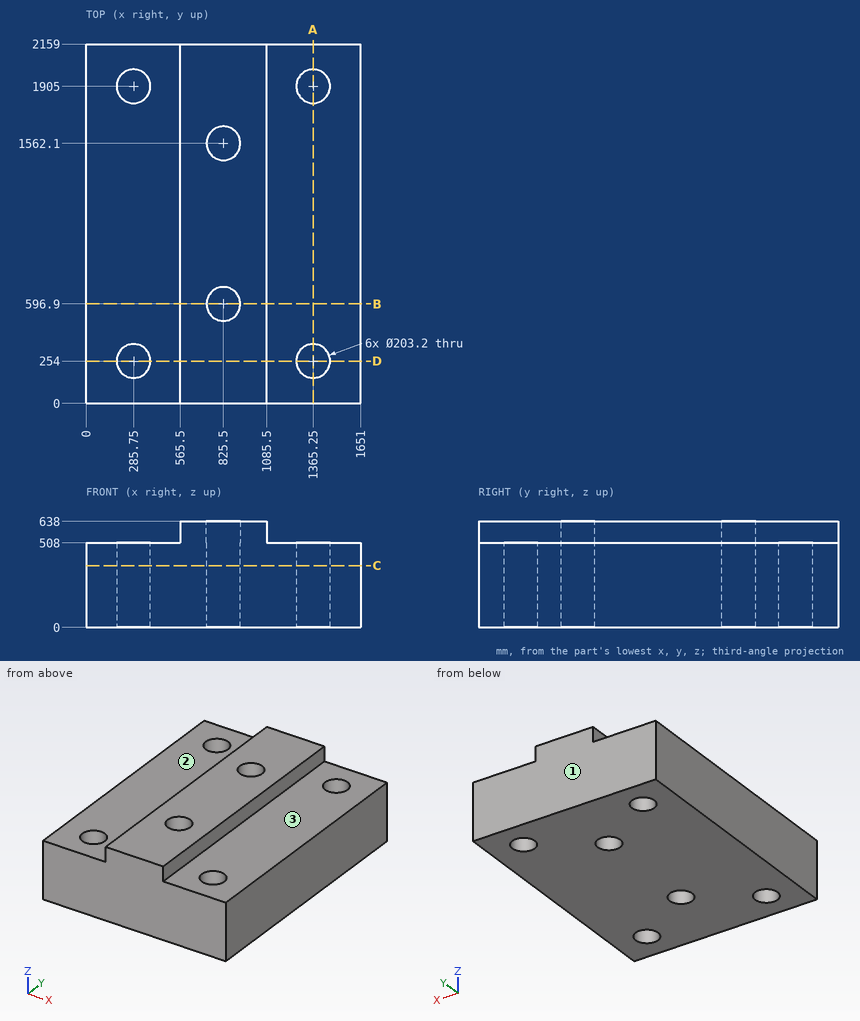
Input: dimensioned drawing with shaded views. Units: mm. Origin: part minimum x, y, z. A direction names the side the tool comes from. Coordinates: 2 decimals unless noted, no trailing zeros. Write each loop counter-clockwise with the first axis right and the second up, starting at its lowest first coordinate (ties: lowest second). Pieces come first, ordered by that corner, then holes. Notation, with made-up numbers: (74.25, 37) -> (106.25, 37) arc R10 ccw to (106.25, 49) -> close; hole circle Ø7 at (87.25, 39.25). An arc over 180 degrees is marked (long way). Return JSON: item names as keys, results as strings. Group by question number.
1) Section query D-D, the plane y = 254. Return loops of the section in (x, z).
2) Set-up query: the marked faces 1, 2 and 3. Return all of +Z, -Z, +X, -X, +Y, -Y with unobstructed straight access to the full face (end or side cutting, diameter ignored); none if empty.
3) Section query A-A, the plane x = 1365.25. Return loops of the section in (y, z).
4) Section query B-B, the plane y = 596.9. Return loops of the section in (x, z), plus the area to 3 significant figures.
5) Ray query, line 1 along Y through (x, z) = (1365.25, 301); line 2 along X through (y, z) = (1905, 295.5); line 3 along Y through (x, z) = (825.5, 284.5). Return the intervals inside material, ascending.
6) Section query C-C, the plane z = 372. Return loops of the section in (x, y), plus the area to 3 significant figures.
From the geometry:
{
 "1": {"outline": "(0, 0) -> (184.15, 0) -> (184.15, 508) -> (0, 508) -> close; (387.35, 0) -> (1263.65, 0) -> (1263.65, 508) -> (1085.5, 508) -> (1085.5, 638) -> (565.5, 638) -> (565.5, 508) -> (387.35, 508) -> close; (1466.85, 0) -> (1651, 0) -> (1651, 508) -> (1466.85, 508) -> close"},
 "2": {"face 1": "+Z, -Z, +X, -X, +Y", "face 2": "+Z, -X, +Y, -Y", "face 3": "+Z, +X, +Y, -Y"},
 "3": {"outline": "(0, 0) -> (152.4, 0) -> (152.4, 508) -> (0, 508) -> close; (355.6, 0) -> (1803.4, 0) -> (1803.4, 508) -> (355.6, 508) -> close; (2006.6, 0) -> (2159, 0) -> (2159, 508) -> (2006.6, 508) -> close"},
 "4": {"outline": "(0, 0) -> (723.9, 0) -> (723.9, 638) -> (565.5, 638) -> (565.5, 508) -> (0, 508) -> close; (927.1, 0) -> (1651, 0) -> (1651, 508) -> (1085.5, 508) -> (1085.5, 638) -> (927.1, 638) -> close", "area": "777,000 mm²"},
 "5": {"line 1": "0 to 152.4, 355.6 to 1803.4, 2006.6 to 2159", "line 2": "0 to 184.15, 387.35 to 1263.65, 1466.85 to 1651", "line 3": "0 to 495.3, 698.5 to 1460.5, 1663.7 to 2159"},
 "6": {"outline": "(0, 0) -> (1651, 0) -> (1651, 2159) -> (0, 2159) -> close; hole circle Ø203.2 at (285.75, 254); hole circle Ø203.2 at (285.75, 1905); hole circle Ø203.2 at (825.5, 596.9); hole circle Ø203.2 at (825.5, 1562.1); hole circle Ø203.2 at (1365.25, 254); hole circle Ø203.2 at (1365.25, 1905)", "area": "3,370,000 mm²"}
}
